Geometry: final body of the model. Coordinates: model frame, mm. A direction names the side the tool comes from. Give positions to 0.01 mm unless a question says otherwise; leave off trailing zeros. Order: outer loops, then holes, each group sorted by start corner. A loop starts at its lowest first (then second) coordinate and runs counter-clockwise, first axis right, second up. Notation, with made-up numbers: (49, 56) - (94, 56) arc R7 cw to (94, 68) - close; hole circle Ø7 at (51.25, -24). An arc over 180 degrees is marked (long way). Write item = value, one per line. Start each with the question number.
from build123d import *
from OCP.BRepFilletAPI import BRepFilletAPI_MakeChamfer

# Parameters (mm, degrees)
SKETCH_1_R          = 2.1
SKETCH_1_R_2        = 10.5
SKETCH_1_R_3        = 10
EXTRUDE_1_DEPTH     = 4
CHAMFER_1_SIZE      = 5
FILLET_1_R          = 10
SKETCH_2_R          = 2.1
CUT_EXTRUDE_1_DEPTH = 10
SKETCH_3_R          = 1.6
EXTRUDE_2_DEPTH     = 3
SKETCH_4_R          = 17.6
CUT_EXTRUDE_2_DEPTH = 10
CUT_EXTRUDE_3_DEPTH = 31.8
FILLET_6_R          = 3
FILLET_7_R          = 4
EXTRUDE_START       = -3
EXTRUDE_3_DEPTH     = 3
FILLET_8_R          = 4
CHAMFER_4_SIZE      = 15
CHAMFER_4_SIZE2     = 22.404226252
CUT_EXTRUDE_4_DEPTH = 3
FILLET_11_R         = 5
EXTRUDE_4_DEPTH     = 3
FILLET_12_R         = 5
CHAMFER_5_SIZE      = 1.5
CHAMFER_5_SIZE2     = 1.429177646
CHAMFER_5_SIZE2_2   = 1.610271544
CUT_EXTRUDE_START   = -10
CUT_EXTRUDE_5_DEPTH = 10


with BuildPart() as part:
    # 草图1 → 凸台-拉伸1 (new body)
    with BuildSketch(Plane(origin=(0, 0, 0), x_dir=(1, 0, 0), z_dir=(0, 1, 0))):
        Polygon((0, 31.819805153), (-31.819805153, 0), (0, -31.819805153), (15.909902577, -15.909902577), (67.5, -15.909902577), (67.5, -22.5), (112.5, -22.5), (112.5, 22.5), (67.5, 22.5), (67.5, 15.909902577), (15.909902577, 15.909902577), align=None)
        with Locations(Location((0, 14, 0), (0, 0, 270))):
            Circle(SKETCH_1_R, mode=Mode.SUBTRACT)
        with Locations(Location((14, 0, 0), (0, 0, 270))):
            Circle(SKETCH_1_R, mode=Mode.SUBTRACT)
        with Locations(Location((0, -14, 0), (0, 0, 270))):
            Circle(SKETCH_1_R, mode=Mode.SUBTRACT)
        with Locations(Location((-14, 0, 0), (0, 0, 270))):
            Circle(SKETCH_1_R, mode=Mode.SUBTRACT)
        with Locations(Location((90, 0, 0), (0, 0, 270))):
            Circle(SKETCH_1_R_2, mode=Mode.SUBTRACT)
        with Locations(Location((0, 22.5, 0), (0, 0, 270))):
            Circle(SKETCH_1_R, mode=Mode.SUBTRACT)
        with Locations(Location((0, -22.5, 0), (0, 0, 270))):
            Circle(SKETCH_1_R, mode=Mode.SUBTRACT)
        with Locations(Location((0, 0, 0), (0, 0, 270))):
            Circle(SKETCH_1_R_3, mode=Mode.SUBTRACT)
        with Locations(Location((-22.5, 0, 0), (0, 0, 270))):
            Circle(SKETCH_1_R, mode=Mode.SUBTRACT)
    extrude(amount=EXTRUDE_1_DEPTH)

    # 倒角1
    chamfer_1_edges = [part.edges().sort_by_distance(p)[0] for p in [
        (112.5, 2, -22.5),
        (112.5, 2, 22.5),
        (0, 2, 31.819805153),
        (-31.819805153, 2, 0),
        (0, 2, -31.819805153),
    ]]
    chamfer(chamfer_1_edges, length=CHAMFER_1_SIZE)

    # 圆角1
    # the kernel refuses this fillet: 10 mm, written as the material it adds along each edge
    with BuildSketch(Plane(origin=(15.909902577, 0, -15.909902577), x_dir=(-0.707106781186552, 0, -0.707106781186543), z_dir=(0, 1, 0))) as fillet_1_piece_1:
        with BuildLine():
            CenterArc((FILLET_1_R * 0.414213562373, -FILLET_1_R), FILLET_1_R, 90, 45)
            Line((-FILLET_1_R * 0.292893218813, -FILLET_1_R * 0.292893218813), (-FILLET_1_R * 0.307035354437, -FILLET_1_R * 0.27875108319))
            Line((-FILLET_1_R * 0.307035354437, -FILLET_1_R * 0.27875108319), (-FILLET_1_R * 0.00828427124746, FILLET_1_R * 0.02))
            Line((-FILLET_1_R * 0.00828427124746, FILLET_1_R * 0.02), (FILLET_1_R * 0.414213562373, FILLET_1_R * 0.02))
            Line((FILLET_1_R * 0.414213562373, FILLET_1_R * 0.02), (FILLET_1_R * 0.414213562373, 0))
        make_face()
    extrude(amount=4)
    with BuildSketch(Plane(origin=(15.909902577, 0, 15.909902577), x_dir=(-0.7071067811865422, 0, 0.707106781186553), z_dir=(0, 1, 0))) as fillet_1_piece_2:
        with BuildLine():
            CenterArc((FILLET_1_R * 0.414213562373, FILLET_1_R), FILLET_1_R, 225, 45)
            Line((-FILLET_1_R * 0.292893218813, FILLET_1_R * 0.292893218813), (-FILLET_1_R * 0.307035354437, FILLET_1_R * 0.27875108319))
            Line((-FILLET_1_R * 0.307035354437, FILLET_1_R * 0.27875108319), (-FILLET_1_R * 0.00828427124746, -FILLET_1_R * 0.02))
            Line((-FILLET_1_R * 0.00828427124746, -FILLET_1_R * 0.02), (FILLET_1_R * 0.414213562373, -FILLET_1_R * 0.02))
            Line((FILLET_1_R * 0.414213562373, -FILLET_1_R * 0.02), (FILLET_1_R * 0.414213562373, 0))
        make_face()
    extrude(amount=4)
    with BuildSketch(Plane(origin=(67.5, 0, 15.909902577), x_dir=(-1, 0, 0), z_dir=(0, 1, 0))) as fillet_1_piece_3:
        with BuildLine():
            CenterArc((9.400668296, 10), FILLET_1_R, 199.937217397, 70.062782603)
            Line((0, 6.590097423), (-0.188013366, 6.521899372))
            ThreePointArc((-0.188013366, 6.521899372), (-0.2, 3.295048712), (-0.2, 0))
            Line((-0.2, 0), (0, -0.2))
            Line((0, -0.2), (9.400668296, -0.2))
            Line((9.400668296, -0.2), (9.400668296, 0))
        make_face()
    extrude(amount=4)
    with BuildSketch(Plane(origin=(67.5, 0, -15.909902577), x_dir=(-1, 0, 0), z_dir=(0, 1, 0))) as fillet_1_piece_4:
        with BuildLine():
            CenterArc((9.400668296, -10), FILLET_1_R, 90, 70.062782603)
            Line((0, -6.590097423), (-0.188013366, -6.521899372))
            ThreePointArc((-0.188013366, -6.521899372), (-0.2, -3.295048712), (-0.2, 0))
            Line((-0.2, 0), (0, 0.2))
            Line((0, 0.2), (9.400668296, 0.2))
            Line((9.400668296, 0.2), (9.400668296, 0))
        make_face()
    extrude(amount=4)

    # 草图2 → 切除-拉伸1 (cut)
    with BuildSketch(Plane.XZ):
        with Locations(Location((106.464466094, 16.464466094, 0), (0, 0, 270))):
            Circle(SKETCH_2_R)
        with Locations(Location((106.464466094, -16.464466094, 0), (0, 0, 270))):
            Circle(SKETCH_2_R)
        with Locations(Location((73.535533906, -16.464466094, 0), (0, 0, 90))):
            Circle(SKETCH_2_R)
        with Locations(Location((73.535533906, 16.464466094, 0), (0, 0, 90))):
            Circle(SKETCH_2_R)
        with Locations(Location((24.075684952, 10.909902577, 0), (0, 0, 270))):
            Circle(SKETCH_2_R)
        with Locations(Location((59.075684952, 10.909902577, 0), (0, 0, 270))):
            Circle(SKETCH_2_R)
        with Locations(Location((59.075684952, -10.909902577, 0), (0, 0, 90))):
            Circle(SKETCH_2_R)
        with Locations(Location((24.075684952, -10.909902577, 0), (0, 0, 90))):
            Circle(SKETCH_2_R)
    extrude(amount=-CUT_EXTRUDE_1_DEPTH, mode=Mode.SUBTRACT)

    # 草图3 → 凸台-拉伸2 (add)
    with BuildSketch(Plane(origin=(0, 4, 0), x_dir=(1, 0, 0), z_dir=(0, 1, 0))):
        Polygon((74.689031721, 83.86671265), (39.075684952, 15.909902577), (49.236670423, 15.909902577), (78, 70.795621063), (98.581853944, 22.5), (107.5, 22.5), (81.347717681, 83.86671265), align=None)
        with Locations(Location((78, 77.942286341, 0), (0, 0, 270))):
            Circle(SKETCH_3_R, mode=Mode.SUBTRACT)
    extrude(amount=-EXTRUDE_2_DEPTH)

    # 草图4 → 切除-拉伸2 (cut)
    with BuildSketch(Plane(origin=(0, 4, 0), x_dir=(1, 0, 0), z_dir=(0, 1, 0))):
        with Locations(Location((0, 0, 0), (0, 0, 270))):
            Circle(SKETCH_4_R)
    extrude(amount=-CUT_EXTRUDE_2_DEPTH, mode=Mode.SUBTRACT)

    # 草图5 → 切除-拉伸3 (cut)
    with BuildSketch(Plane(origin=(0, 4, 0), x_dir=(1, 0, 0), z_dir=(0, 1, 0))):
        with BuildLine():
            Line((24.075684952, 3.202114308), (24.075684952, -3.202114308))
            ThreePointArc((24.075684952, -3.202114308), (28.335182293, -4.485987695), (31.175684952, -7.909902577))
            Line((31.175684952, -7.909902577), (51.975684952, -7.909902577))
            ThreePointArc((51.975684952, -7.909902577), (54.816187611, -4.485987695), (59.075684952, -3.202114308))
            Line((59.075684952, -3.202114308), (59.075684952, 3.202114308))
            ThreePointArc((59.075684952, 3.202114308), (54.816187611, 4.485987695), (51.975684952, 7.909902577))
            Line((51.975684952, 7.909902577), (31.175684952, 7.909902577))
            ThreePointArc((31.175684952, 7.909902577), (28.335182293, 4.485987695), (24.075684952, 3.202114308))
        make_face()
    extrude(amount=-CUT_EXTRUDE_3_DEPTH, mode=Mode.SUBTRACT)

    # 圆角6
    fillet_6_edges = [part.edges().sort_by_distance(p)[0] for p in [
        (24.075684952, 2, -3.202114308),
        (31.175684952, 2, -7.909902577),
        (51.975684952, 2, -7.909902577),
        (59.075684952, 2, -3.202114308),
        (59.075684952, 2, 3.202114308),
        (51.975684952, 2, 7.909902577),
        (31.175684952, 2, 7.909902577),
        (24.075684952, 2, 3.202114308),
    ]]
    fillet(fillet_6_edges, radius=FILLET_6_R)

    # 圆角7
    fillet_7_edges = [part.edges().sort_by_distance(p)[0] for p in [
        (49.236670423, 2.5, -15.909902577),
    ]]
    fillet(fillet_7_edges, radius=FILLET_7_R)

    # 草图6 → 凸台-拉伸3 (add)
    with BuildSketch(Plane(origin=(0, 4, 0), x_dir=(1, 0, 0), z_dir=(0, 1, 0)).offset(EXTRUDE_START)):
        with BuildLine():
            Line((67.5, 22.5), (52.690267267, 22.5))
            Line((52.690267267, 22.5), (52.305934696, 21.766622828))
            ThreePointArc((52.305934696, 21.766622828), (52.426407737, 17.83950177), (55.848898132, 15.909902577))
            Line((55.848898132, 15.909902577), (58.099331704, 15.909902577))
            ThreePointArc((58.099331704, 15.909902577), (63.839583189, 17.721525883), (67.5, 22.5))
        make_face()
    extrude(amount=EXTRUDE_3_DEPTH)

    # 圆角8
    fillet_8_edges = [part.edges().sort_by_distance(p)[0] for p in [
        (98.581853944, 2.5, -22.5),
        (78, 2.5, -70.795621063),
        (52.690267267, 2.5, -22.5),
    ]]
    fillet(fillet_8_edges, radius=FILLET_8_R)

    # 倒角4
    chamfer_4_edges = [part.edges().sort_by_distance(p)[0] for p in [
        (39.075684952, 2.5, -15.909902577),
    ]]
    chamfer_4_side = [part.faces().sort_by_distance(p)[0] for p in [
        (33.368590927, 1.7, -15.909902577),
    ]]
    chamfer(chamfer_4_edges, length=CHAMFER_4_SIZE, length2=CHAMFER_4_SIZE2, reference=chamfer_4_side[0])

    # 草图7 → 切除-拉伸4 (cut)
    with BuildSketch(Plane(origin=(0, 4, 0), x_dir=(1, 0, 0), z_dir=(0, 1, 0))):
        with BuildLine():
            Line((32.197031179, 15.909902577), (56.151580128, 15.909902577))
            Line((56.151580128, 15.909902577), (59.302494975, 17.5))
            ThreePointArc((59.302494975, 17.5), (51.509584112, 21.997718325), (51.505632804, 30.995435494))
            Line((51.505632804, 30.995435494), (32.197031179, 15.909902577))
        make_face()
    extrude(amount=-CUT_EXTRUDE_4_DEPTH, mode=Mode.SUBTRACT)

    # 圆角11
    fillet_11_edges = [part.edges().sort_by_distance(p)[0] for p in [
        (49.475280099, 2.5, -35.754241184),
        (24.075684952, 2.5, -15.909902577),
    ]]
    fillet(fillet_11_edges, radius=FILLET_11_R)

    # 草图8 → 凸台-拉伸4 (add)
    with BuildSketch(Plane(origin=(0, 4, 0), x_dir=(1, 0, 0), z_dir=(0, 1, 0))):
        Polygon((81.347717681, 83.86671265), (83.347717681, 83.86671265), (85.253411001, 74.701946198), align=None)
        Polygon((74.689031721, 83.86671265), (72.689031721, 83.86671265), (69.886157582, 74.701946198), align=None)
    extrude(amount=-EXTRUDE_4_DEPTH)

    # 圆角12
    fillet_12_edges = [part.edges().sort_by_distance(p)[0] for p in [
        (85.253411001, 2.5, -74.701946198),
        (69.886157582, 2.5, -74.701946198),
    ]]
    fillet(fillet_12_edges, radius=FILLET_12_R)

    # 倒角5: one chamfer whose edges measure the first distance from different faces: ONE call of the kernel's chamfer builder (chamfer() names one face for all edges)
    chamfer_5_edges_1 = [part.edges().sort_by_distance(p)[0] for p in [
        (83.347717681, 2.5, -83.86671265),
    ]]
    chamfer_5_side_1 = [part.faces().sort_by_distance(p)[0] for p in [
        (78.018374701, 2.5, -83.86671265),
    ]]
    chamfer_5_edges_2 = [part.edges().sort_by_distance(p)[0] for p in [
        (72.689031721, 2.5, -83.86671265),
    ]]
    chamfer_5_side_2 = [part.faces().sort_by_distance(p)[0] for p in [
        (71.355755289, 2.5, -79.50719934),
    ]]
    chamfer_5 = BRepFilletAPI_MakeChamfer(part.part.solid().wrapped)
    for e in chamfer_5_edges_1:
        chamfer_5.Add(CHAMFER_5_SIZE, CHAMFER_5_SIZE2, e.wrapped, chamfer_5_side_1[0].wrapped)  # the first distance lies on this face
    for e in chamfer_5_edges_2:
        chamfer_5.Add(CHAMFER_5_SIZE, CHAMFER_5_SIZE2_2, e.wrapped, chamfer_5_side_2[0].wrapped)  # the first distance lies on this face
    add(Compound.cast(chamfer_5.Shape()), mode=Mode.REPLACE)

    # 草图9 → 切除-拉伸5 (cut)
    with BuildSketch(Plane(origin=(0, 4, 0), x_dir=(1, 0, 0), z_dir=(0, 1, 0)).offset(CUT_EXTRUDE_START)):
        with BuildLine():
            Line((22.354046886, 15.909902577), (58.099331704, 15.909902577))
            ThreePointArc((58.099331704, 15.909902577), (63.839583189, 17.721525883), (67.5, 22.5))
            Line((67.5, 22.5), (112.713100818, 22.5))
            Line((112.713100818, 22.5), (128.205404221, 15.909902577))
            Line((128.205404221, 15.909902577), (92.949872776, 93.149070556))
            Line((92.949872776, 93.149070556), (54.968117123, 93.149070556))
            Line((54.968117123, 93.149070556), (22.354046886, 15.909902577))
        make_face()
    extrude(amount=CUT_EXTRUDE_5_DEPTH, mode=Mode.SUBTRACT)


solid = part.part
Q1. Section C-C, the plane y = 0.7. Count the separate pieces of the cut face and the enclosed holes in it, then the cut area to 3 significant figures.
Q2. Section B-B, the plane x = -22.5. Return the cut outline in (y, z), then the cut area to 3 significant figures.
Q3. Pull-direction query (X, two-part tool) for faces 4 (the flat face through (0, 2, -28.284)), 5 (the cylindrical face through (-0.8, 1.97, -20.56)), 6 (the flat face through (-28.284, 2, 0)); classes: +X half, -X half, draft (parallel to the pull), parting line (faces both ways), or undercut.
Q4. Contact query for flat-ended pins moving along their axis: pin 1 (5 mm diameter, centred on x = 106.46, z = -16.46, fed in from -Y); pin 2 (2 mm diameter, centred on x = 19, z = -17.5, fed in from +Y); pin 3 (2 mm diameter, centred on x = 39, y = 1.5, fed in from +Z). Output: stop coordinate, or through.
Q5. Section A-A, the plane x = 41.5. Return the cut outline in (y, z), then the cut area to 3 significant figures.
Q6. Set-up query: faces 1 (the cylindrical face through (31.52, 1.97, 7.55)), 2 (the flat face through (8.19, 1.97, 23.63)), 3 (the flat face through (88, 2, -22.5)). Return all of +Z, -Z, +X, -X, +Y, -Y with unobstructed straight access to the full face (end or side cutting, diameter ignored); none if empty.
Q7. Material intervals for line 1 along X through (y, z) = (2.7, 0); line 2 along Z through (x, y) = (73.5, 2.3); line 3 along Z through (x, y) = (47.5, 3.8), sorted ascending. Write a range as from..to.
The answers:
q1.separate_pieces = 1
q1.enclosed_holes = 14
q1.area = 3,490 mm²
q2.outline = (0, -9.32) - (4, -9.32) - (4, -2.1) - (0, -2.1) - close; (0, 2.1) - (4, 2.1) - (4, 9.32) - (0, 9.32) - close
q2.area = 57.8 mm²
q3.face_4 = draft
q3.face_5 = undercut
q3.face_6 = -X half
q4.pin_1 = 0
q4.pin_2 = through
q4.pin_3 = 15.91
q5.outline = (0, -15.91) - (4, -15.91) - (4, -7.91) - (0, -7.91) - close; (0, 7.91) - (4, 7.91) - (4, 15.91) - (0, 15.91) - close
q5.area = 64.0 mm²
q6.face_1 = +Y, -Y
q6.face_2 = +Z, +Y, -Y
q6.face_3 = -Z, +X, +Y, -Y
q7.line_1 = -28.28..-24.6, -20.4..-17.6, 17.6..24.08, 59.08..79.5, 100.5..112.5
q7.line_2 = -22.5..-18.56, -14.36..14.36, 18.56..22.5
q7.line_3 = -15.91..-7.91, 7.91..15.91
